For this review, use the dimensioned drawing (mm, ordinates from the lowest corner) and the shaded views. A direction names the side the tool comes from. Coordinates: 2 decimals unless noted, no trailing zeros. Order: outer loops, then holes, each group sorted by start corner. A loop starts at its lowest first (then second) coordinate and runs counter-clockwise, first axis right, second up. Notation, with made-up numbers: M 56.5,8.5 L 65.5,8.5 A24 ccw 65.5,20.5 Z; hole C 66.25,-26.5 d8. An arc over 180 degrees is marked long. Answer in a Markdown table with one row per item.
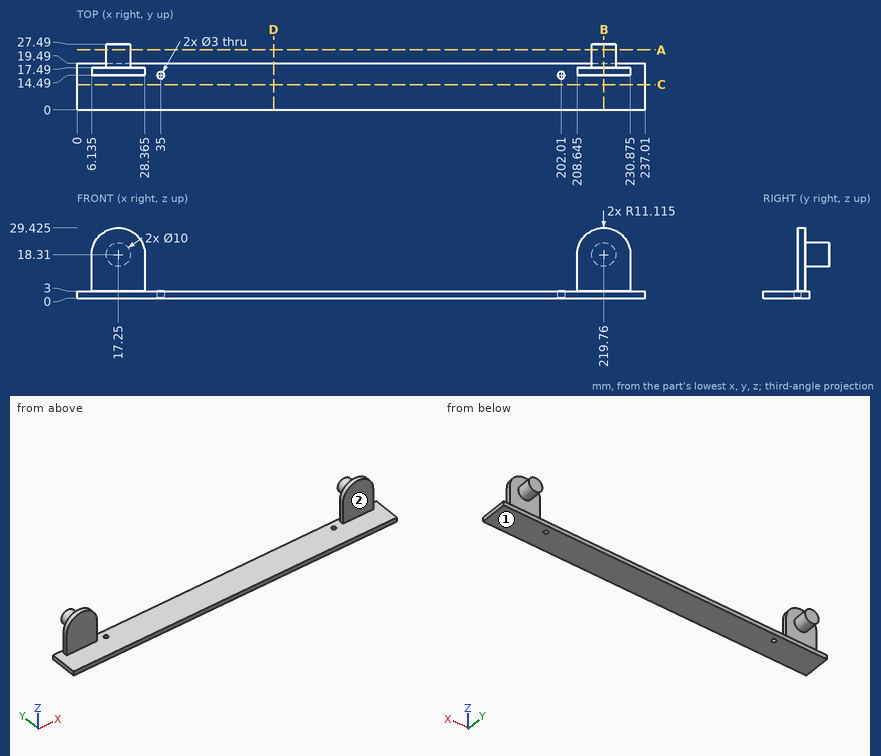
(1) Insertion check: pin 1 Ø10 at (x, y) = (162, 17.5) entering from +Z; pin 2 Ø10 at (y, z) = (19.5, 20.5) entering from -X (3 decimals); pin 3 Ø2.5 at (y, z) = (15.5, 9.5) entering from +X (3 decimals). Each pin has a flat end and moves straight along its axis. Give the tip position at first contact, or say it passes through.
Return value:
| item | result |
|---|---|
| pin 1 | stops at z = 3 |
| pin 2 | stops at x = 6.135 |
| pin 3 | stops at x = 230.875 |
(2) Add section D-D, the plane x = 82. Give the boundary of the cut face in (y, z), and give its area (3 significant figures).
Return value:
| item | result |
|---|---|
| outline | M 0,0 L 19.49,0 L 19.49,3 L 0,3 Z |
| area | 58.5 mm2 |
(3) For line 1 along Y through (x, z) = (202.01, 0.85); line 2 along Z through (x, y) = (27, 11.25); line 3 along Y through (x, z) = (226, 25), list the stretches that pass through material, from the lowest coordinate up. Write a range as from..to.
Return value:
| item | result |
|---|---|
| line 1 | y = 0..12.99, 15.99..19.49 |
| line 2 | z = 0..3 |
| line 3 | y = 14.49..17.49 |
(4) Add section C-C, the plane y = 10.5. Give the boundary of the cut face in (x, z).
Return value:
| item | result |
|---|---|
| outline | M 0,0 L 237.01,0 L 237.01,3 L 0,3 Z |
(5) For the marked faces 1 and 2, list the 3-axis set-ups (+Z, -Z, +X, -X, +Y, -Y) from which the entire face can be reached by the end or side of a thin tool; tool diameter is ignored.
Return value:
| item | result |
|---|---|
| face 1 | -Z, +X, -X, +Y, -Y |
| face 2 | +Z, +X, -X, -Y |
(6) Add section A-A, the plane y = 25. Give the boundary of the cut face in (x, z), and give its area (3 significant figures).
Return value:
| item | result |
|---|---|
| outline | C 17.25,18.31 d10; C 219.76,18.31 d10 |
| area | 157 mm2 |
(7) Add section B-B, the plane x = 219.76. Give the boundary of the cut face in (y, z) (3 decimals).
Return value:
| item | result |
|---|---|
| outline | M 0,0 L 19.49,0 L 19.49,3 L 17.49,3 L 17.49,13.31 L 27.49,13.31 L 27.49,23.31 L 17.49,23.31 L 17.49,29.425 L 14.49,29.425 L 14.49,3 L 0,3 Z |
